Work out the finished part from the listing and answer in its coordinate system (mm). Round coordinates to 2 decimals unless told otherwise and drop trailing zeros. Write each loop counter-clockwise with the first axis right and the second up, starting at its lowest first coordinate (ties: lowest second). Pieces come first, ordered by that corner, then holes.
1. Find section B-B (z = 1.5). Write down the section's boundary in (x, y).
2. Find section C-C (x = -47.5). Write down the section's boundary in (y, z), and give its area (3 significant figures).
3. Straight lines are drawn through the part: probe 1 along X at (y, z) = (-7, 6.5); probe 2 along Y at (x, z) = (22.5, 2); probe 3 along Y at (x, z) = (-87.5, 5.25). For each, find the intervals that lie inside material, in ascending order.
4. Find section D-D (y = 15). Write down the section's boundary in (x, z), and give its area (3 significant figures).
5. Find section A-A (x = -87.5). Write down the section's boundary in (y, z), and give its area (3 significant figures).
6. Flat-ended cylindrical pins translate along their axes: pin 1 Ø1.5 at (x, z) = (-45.5, 1.5) entering from -Y; pin 2 Ø11.5 at (x, y) = (-32.5, -8.52) entering from -Z; pin 3 Ø3 at (y, z) = (8, 8) entering from +X; pin 4 Ø4 at (x, y) = (49.5, -12) entering from -Z. Find the tip coordinate at first contact, or state that the pin passes through.
7. Determine the mould class of faces 1 (the face through (79.96, -14.3, 4.56)), 2 (the face through (-2, 26.98, 4)), 3 (the face through (26.88, -16.95, 4.56)), 4 (the face through (-0.5, -21.2, 3)) for opening direction Y: pulls with the +Y half, pulls with the -Y half, needs draft (parallel to the pull), parting line crosses it, or undercut.
```python
from build123d import *

# Parameters (mm, degrees)
SKETCH1_W           = 226
SKETCH1_H           = 53
BOSS_EXTRUDE1_DEPTH = 9
SKETCH3_R           = 9.5
CUT_EXTRUDE1_DEPTH  = 9
SKETCH2_W           = 11
SKETCH2_H           = 3
CUT_EXTRUDE2_DEPTH  = 54
SKETCH4_W           = 3
SKETCH4_H           = 5
CUT_EXTRUDE3_DEPTH  = 227


with BuildPart() as part:
    # Sketch1 → Boss-Extrude1 (new body)
    with BuildSketch(Plane.XY):
        with Locations((0, 0.4802203)):
            Rectangle(SKETCH1_W, SKETCH1_H)
    extrude(amount=BOSS_EXTRUDE1_DEPTH)

    # Sketch3 → Cut-Extrude1 (cut)
    with BuildSketch(Plane.XY.offset(9)):
        with Locations((-87.5, -8.5197797)):
            Circle(SKETCH3_R)
        with Locations((-32.5, -8.5197797)):
            Circle(SKETCH3_R)
        with Locations((22.5, -8.5197797)):
            Circle(SKETCH3_R)
        with Locations((87.5, -8.5197797)):
            Circle(SKETCH3_R)
    extrude(amount=-CUT_EXTRUDE1_DEPTH, mode=Mode.SUBTRACT)

    # Sketch2 → Cut-Extrude2 (cut, through all)
    with BuildSketch(Plane.XZ.offset(26.0197797)):
        with Locations((-107.5, 7.5)):
            Rectangle(SKETCH2_W, SKETCH2_H)
        with Locations((-107.5, 1.5)):
            Rectangle(SKETCH2_W, SKETCH2_H)
        with Locations((107.5, 7.5)):
            Rectangle(SKETCH2_W, SKETCH2_H)
        with Locations((107.5, 1.5)):
            Rectangle(SKETCH2_W, SKETCH2_H)
    extrude(amount=-CUT_EXTRUDE2_DEPTH, mode=Mode.SUBTRACT)

    # Sketch4 → Cut-Extrude3 (cut, through all)
    with BuildSketch(Plane.ZY.offset(113)):
        Polygon((0, -21.0197797), (0, -26.0197797), (3, -26.0197797), (3, -23.123504735), (3, -21.0197797), align=None)
        with Locations((7.5, -23.5197797)):
            Rectangle(SKETCH4_W, SKETCH4_H)
    extrude(amount=-CUT_EXTRUDE3_DEPTH, mode=Mode.SUBTRACT)


solid = part.part
```
Worked answers:
1. outline: (-102, -21.02) - (102, -21.02) - (102, 26.98) - (-102, 26.98) - close; hole circle Ø19 at (-87.5, -8.52); hole circle Ø19 at (-32.5, -8.52); hole circle Ø19 at (22.5, -8.52); hole circle Ø19 at (87.5, -8.52)
2. outline: (-26.02, 3) - (-21.02, 3) - (-21.02, 0) - (26.98, 0) - (26.98, 9) - (-21.02, 9) - (-21.02, 6) - (-26.02, 6) - close
2. area: 447 mm2
3. probe 1: x = -102 to -96.88, -78.12 to -41.88, -23.12 to 13.12, 31.88 to 78.12, 96.88 to 102
3. probe 2: y = -21.02 to -18.02, 0.98 to 26.98
3. probe 3: y = -26.02 to -18.02, 0.98 to 26.98
4. outline: (-113, 3) - (-102, 3) - (-102, 0) - (102, 0) - (102, 3) - (113, 3) - (113, 6) - (102, 6) - (102, 9) - (-102, 9) - (-102, 6) - (-113, 6) - close
4. area: 1,900 mm2
5. outline: (-26.02, 3) - (-21.02, 3) - (-21.02, 0) - (-18.02, 0) - (-18.02, 9) - (-21.02, 9) - (-21.02, 6) - (-26.02, 6) - close; (0.98, 0) - (26.98, 0) - (26.98, 9) - (0.98, 9) - close
5. area: 276 mm2
6. pin 1: stops at y = -21.02
6. pin 2: passes through
6. pin 3: stops at x = 102
6. pin 4: stops at z = 0
7. face 1: undercut
7. face 2: pulls with the +Y half
7. face 3: undercut
7. face 4: needs draft
